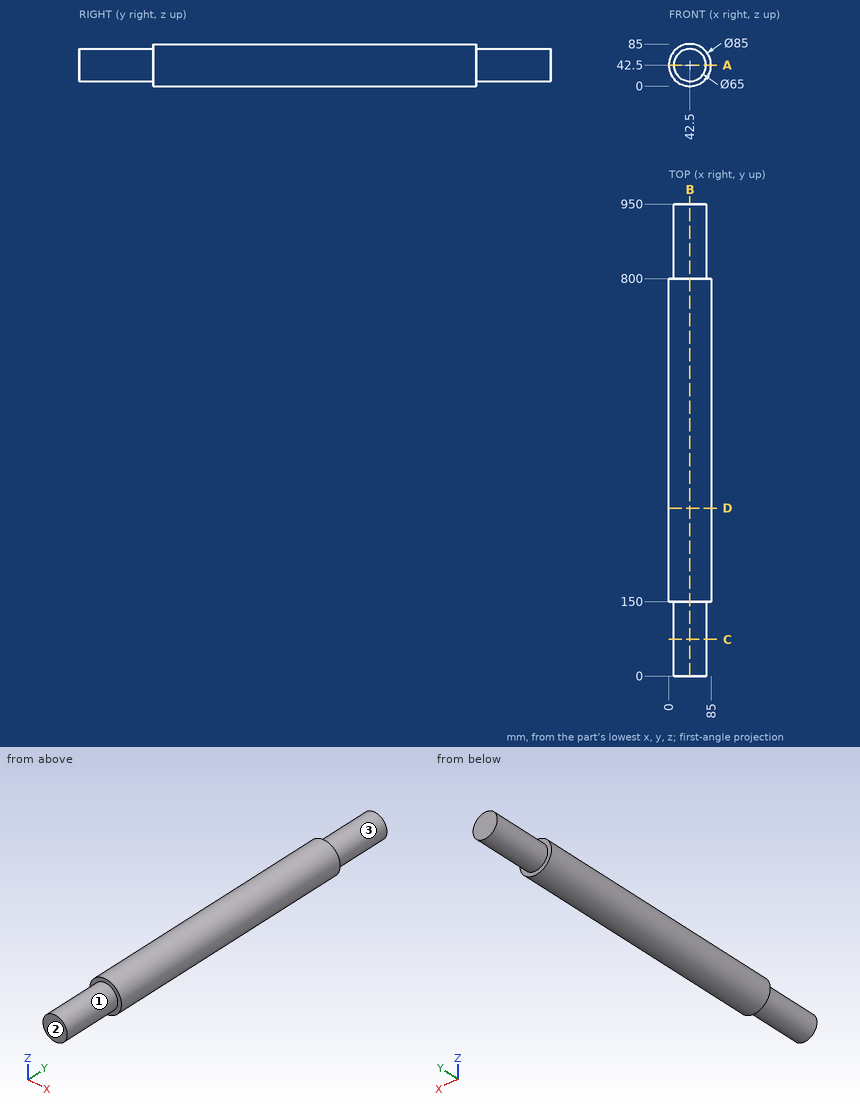
Design review of the part shown in the three views and the two pictorial views. Dimensions are in mm from the part's minimum x, y and z. A direction names the side the tool comes from. Round coordinates to 2 decimals unless told otherwise and drop trailing zeros. Loops run counter-clockwise (first coordinate to the right, second up) from the corner with the lowest first, then second, coordinate; pieces in that order, holes last. Notation, with made-up numbers: (-24.5, 15) - (-10.5, 15) arc R6 ccw to (-10.5, 21) - close; hole circle Ø7 at (33, 36.25). An arc over 180 degrees is marked (long way). Use CSV: the item, a comma, the result in double quotes.
(1) Take a section at B-B, the plane x = 42.5. Give the boundary of the cut face in (y, z).
Working result:
outline,"(0, 10) - (150, 10) - (150, 0) - (800, 0) - (800, 10) - (950, 10) - (950, 75) - (800, 75) - (800, 85) - (150, 85) - (150, 75) - (0, 75) - close"
(2) Clearance check with flat-ended pins moving along their axes: P1, Ø8, axis at x = 46, y = 187.5, coming from the -Z side; P2, Ø6, axis at y = 339.5, z = 15.5, coming from the -X side; P3, Ø4, axis at y = 335, z = 61, coming from the -X side. State where each tip first meets the part, or that it passes through.
Working result:
P1,"stops at z = 0"
P2,"stops at x = 7.43"
P3,"stops at x = 3.33"
(3) Take a section at C-C, the plane y = 73.5. Give the boundary of the cut face in (x, z), plus the area to 3 significant figures.
Working result:
outline,"circle Ø65 at (42.5, 42.5)"
area,"3,320 mm^2"
(4) Machinability: for the marked faces 1, 2 and 3, which of the approach directions +Z, -Z, +X, -X, +Y, -Y give a long, thin tool a straight path to every point of the face, cutting with its end or side? Answer none if there is none.
Working result:
face 1,"-Y"
face 2,"+Z, -Z, +X, -X, -Y"
face 3,"+Y"
(5) Take a section at D-D, the plane y = 338. Give the boundary of the cut face in (x, z).
Working result:
outline,"circle Ø85 at (42.5, 42.5)"
(6) Take a section at A-A, the plane z = 42.5. Give the boundary of the cut face in (x, y), plus the area to 4 significant figures.
Working result:
outline,"(0, 150) - (10, 150) - (10, 0) - (75, 0) - (75, 150) - (85, 150) - (85, 800) - (75, 800) - (75, 950) - (10, 950) - (10, 800) - (0, 800) - close"
area,"74,750 mm^2"
(7) For line 1 (Y direction, x = 46, z = 6.5); line 2 (X direction, y = 111, z = 20); line 3 (Z direction, x = 66, y = 546), list the stretches that pass through material, from the lowest coordinate up.
Working result:
line 1,"y = 150 to 800"
line 2,"x = 19.05 to 65.95"
line 3,"z = 7.09 to 77.91"
